Part model, mm, in its own coordinate system. Give positions to 0.01 mm unless a question says otherwise; leave off trailing zeros. Write each loop counter-clockwise with the first axis right and the second up, starting at its lowest first coordinate (ties: lowest second). Pieces come first, ordered by that corner, then holes. Notation, with made-up numbers: (74.5, 40) - (91.5, 40) arc R17 cw to (91.5, 68) - close; hole circle Ø5 at (-24.75, -14.75). An arc over 180 degrees is marked (long way). Answer as a JSON object with one key per item and string values. Group by question number.
```python
from build123d import *

# Parameters (mm, degrees)
F2_SIZE = 0.5
F3_SIZE = 0.5


with BuildPart() as f1:
    # F0 (on Right) → F1 (revolve)
    with BuildSketch(Plane.YZ):
        Polygon((25.4, 5), (22.4, 8), (20, 8), (20, 2), (21.453085, 0), (25.4, 0), align=None)
    revolve(axis=Axis((0, 0, 20.029662), (0, 0, 1)))

    # F2
    f2_edges = [f1.edges().sort_by_distance(p)[0] for p in [
        (0, -25.4, 0),
    ]]
    chamfer(f2_edges, length=F2_SIZE)

    # F3
    f3_edges = [f1.edges().sort_by_distance(p)[0] for p in [
        (0, -20, 8),
    ]]
    chamfer(f3_edges, length=F3_SIZE)


solid = f1.part
```
1) Probe line 1 (Y direction, x = 0, z = 3.5); line 2 (X direction, y = 15, z = 6.5). List the from-to ranges inside material, lowest first.
2) Band-saw the part on A-A (y = 0). List the corners of the cut face in (x, z).
3) Band-saw the part on C-C (z = 6.25). List the corners of the cut face in (x, y).
4) Drop flat-ended pins along their axis: P1, Ø1, axis at x = 3.5, z = 5, coming from the -Y side; P2, Ø1.5, axis at y = -20, z = 1, coming from the +X side. Give the stop position or say it passes through.
5) Mould opens along X. For faces 1 (the conical face through (19.613, -4.355, 1.875)), 2 (the flat face through (-19, -11, 0)), 3 (the conical face through (-6.772, 21.505, 7.854)) say: pulls with the +X half, pulls with the -X half, needs draft (parallel to the pull), parting line crosses it, or undercut.
Verdict:
{
 "1": {"line 1": "-25.4 to -20, 20 to 25.4", "line 2": "-18.61 to -13.23, 13.23 to 18.61"},
 "2": {"outline": "(-25.4, 0.5) - (-24.9, 0) - (-21.45, 0) - (-20, 2) - (-20, 7.5) - (-20.5, 8) - (-22.4, 8) - (-25.4, 5) - close; (20, 2) - (21.45, 0) - (24.9, 0) - (25.4, 0.5) - (25.4, 5) - (22.4, 8) - (20.5, 8) - (20, 7.5) - close"},
 "3": {"outline": "circle Ø48.3 at (0, 0); hole circle Ø40 at (0, 0)"},
 "4": {"P1": "y = -25.22", "P2": "x = 16.57"},
 "5": {"face 1": "undercut", "face 2": "needs draft", "face 3": "parting line crosses it"}
}
